Can you work these out from the model? Positions are in its coordinate system, mm. A direction names the side the tool comes from. Give positions to 0.01 mm unless a question says otherwise; leave off trailing zeros. Loops run counter-clockwise (first coordinate to the right, second up) from the corner with the lowest first, then second, coordinate; pieces in that order, holes last.
Solid Edge part; units mm, degrees
sketch "Sketch1" plane through (0, 0, 0) normal (1, 0, 0) x (0, 1, 0)
  arc A0 (2.0255, 64.2182) -> (12.0255, 54.2182) centre (2.0255, 54.2182) cw
  arc A1 (12.0255, 54.2182) -> (62.1552, -15.4154) centre (85.1165, 53.9757) ccw
  arc A2 (62.1552, -15.4154) -> (95.0255, -66.6818) centre (43.6001, -63.4831) cw
  line L0 (95.0255, -66.6818) -> (95.0255, -76.6818)
  line L1 (95.0255, -76.6818) -> (98.0468, -76.6818)
  line L2 (98.0468, -76.6818) -> (98.0468, -65.8944)
  arc A3 (62.6354, -12.4154) -> (98.0468, -65.8944) centre (43.6001, -63.4831) cw
  arc A4 (15.0228, 54.2182) -> (62.6354, -12.4154) centre (85.1165, 53.9757) ccw
  arc A5 (2.0255, 67.2155) -> (15.0228, 54.2182) centre (2.0255, 54.2182) cw
  line L3 (2.0255, 64.2182) -> (2.0255, 67.2155)
  dimension "D1" = 95.0255
  dimension "D2" = 2.0255
extrude "Protrusion1" add sketch "Sketch1" along normal blind 165
sketch "Sketch2" plane through (75, 2.0255, 65.7168) normal (0, -1, 0) x (1, 0, 0)
  line L0 (-75, 1.4986) -> (90, 1.4986)
  line L1 (90, 1.4986) -> (90, -1.4986)
  line L2 (90, -1.4986) -> (-75, -1.4986)
  line L3 (-75, -1.4986) -> (-75, 1.4986)
extrude "Extrusionsausprägung_2" add sketch "Sketch2" along normal blind 56
sketch "Sketch3" plane through (82.5, -22.9745, 67.2155) normal (0, 0, 1) x (0, 1, 0)
  circle A0 centre (-4.5, 42.5) radius 2.25
  circle A1 centre (-4.5, -42.5) radius 2.25
extrude "Cutout1" cut sketch "Sketch3" against normal through all
sketch "Sketch4" plane through (165, 28.0437, -4.7332) normal (1, 0, 0) x (0, 1, 0)
  line L0 (66.9818, -61.9486) -> (63.9818, -61.9486)
  line L1 (63.9818, -61.9486) -> (63.9818, -91.9486)
  line L2 (63.9818, -91.9486) -> (66.9818, -91.9486)
  line L3 (66.9818, -91.9486) -> (66.9818, -61.9486)
  dimension "D1" = 66.9818
  dimension "D2" = 63.9818
extrude "Protrusion2" add sketch "Sketch4" against normal up to vertex (165 mm away)
sketch "Sketch5" plane through (82.5, 95.0255, -86.6818) normal (0, 1, 0) x (1, 0, 0)
  circle A0 centre (-42.5, 0) radius 2.25
  circle A1 centre (42.5, 0) radius 2.25
  dimension "D1" = 42.5
extrude "Cutout2" cut sketch "Sketch5" against normal through all
sketch "Sketch6" plane through (0, 22.0628, -14.7332) normal (-1, 0, 0) x (0, -1, 0)
  line L0 (10.0373, 14.0132) -> (10.0373, 68.9514)
  arc A0 (-42.5155, -1.4376) -> (10.0373, 68.9514) centre (-69.9949, 73.8912) ccw
  line L1 (-42.5155, -1.4376) -> (-37.5155, -1.4376)
  line L2 (10.0373, 14.0132) -> (-37.5155, -1.4376)
  dimension "D1" = 42.5155
  dimension "D2" = 10.0373
extrude "Protrusion3" add sketch "Sketch6" against normal up to vertex (165 mm away)
sketch "Sketch7" plane through (82.5, 16.3444, -2.1232) normal (0, -0.309, -0.9511) x (0, -0.9511, 0.309)
  line L0 (-0.9588, 82.5) -> (-0.9588, 63)
  line L1 (-0.9588, 63) -> (-39.9588, 63)
  line L2 (-39.9588, 63) -> (-39.9588, 82.5)
  line L3 (-39.9588, 82.5) -> (-0.9588, 82.5)
  line L4 (-39.9588, -63) -> (-0.9588, -63)
  line L5 (-0.9588, -63) -> (-0.9588, -82.5)
  line L6 (-0.9588, -82.5) -> (-39.9588, -82.5)
  line L7 (-39.9588, -82.5) -> (-39.9588, -63)
  dimension "D1" = 0.9588
  dimension "D2" = 39.9588
extrude "Extrusionsausschnitt_3" cut sketch "Sketch7" against normal blind 2
sketch "Sketch8" plane through (82.5, 16.3444, -2.1232) normal (0, -0.309, -0.9511) x (0, -0.9511, 0.309)
  line L0 (-30.4588, 63) -> (-10.4588, 63)
  line L1 (-10.4588, 63) -> (-10.4588, 53)
  line L2 (-10.4588, 53) -> (-30.4588, 53)
  line L3 (-30.4588, 53) -> (-30.4588, 63)
  line L4 (-30.4588, -63) -> (-10.4588, -63)
  line L5 (-10.4588, -63) -> (-10.4588, -53)
  line L6 (-10.4588, -53) -> (-30.4588, -53)
  line L7 (-30.4588, -53) -> (-30.4588, -63)
  dimension "D1" = 10.4588
  dimension "D2" = 30.4588
extrude "Extrusionsausschnitt_4" cut sketch "Sketch8" against normal blind 2
sketch "Sketch9" plane through (14.75, 36.4199, -6.5432) normal (0, -0.309, -0.9511) x (1, 0, 0)
  line L0 (14.75, 10) -> (9.75, 10)
  line L1 (9.75, 10) -> (9.75, -10)
  line L2 (9.75, -10) -> (14.75, -10)
  line L3 (14.75, -10) -> (14.75, 10)
  line L4 (120.75, 10) -> (125.75, 10)
  line L5 (125.75, 10) -> (125.75, -10)
  line L6 (125.75, -10) -> (120.75, -10)
  line L7 (120.75, -10) -> (120.75, 10)
extrude "Extrusionsausschnitt_5" cut sketch "Sketch9" against normal blind 56.6903
chamfer "Fase_1" distance 0.5 angle 60 4 edges at (125, -29.7245, 67.2155) (40, -29.7245, 67.2155) (122.75, 95.0255, -86.6818) (37.75, 95.0255, -86.6818) measured on face at (25.85, -44.0812, 67.2154)
properties material "Nylon, allgemein"
(1) Suppose I cut it at D-D on z = 14.5. List the corners of the cut face in (x, y) for me.
Returned:
outline: (0, 12.03) - (165, 12.03) - (165, 27.2) - (0, 27.2) - close
(2) Suppose I cut it at A-A on x = 125. Give the number of separate pieces and of enclosed holes in the cut face, plus the area to 3 significant figures.
Returned:
separate pieces: 3
enclosed holes: 0
area: 1,390 mm2
(3) Thinking about a two-plate mould opening in X: for faces 6 (the cylindrical face through (127.146, 93.107, -87.358)), 7 (the flat face through (145.5, 50, -12)), 8 (the flat face through (81, -26, 67.215)), 9 (the flat face through (19.5, 50, -12)), which applies, pulls with the +X half, pulls with the -X half, needs draft (parallel to the pull), parting line crosses it, or undercut?
Returned:
face 6: undercut
face 7: pulls with the +X half
face 8: needs draft
face 9: pulls with the -X half
(4) Suppose I cut it at B-B on y = -44. List the corners of the cut face in (x, z) for me.
Returned:
outline: (0, 64.22) - (165, 64.22) - (165, 67.22) - (0, 67.22) - close
(5) Will these pins go through, and if not, where does the flat tip stop? P1, Ø16, axis at x = 112, z = -89, coming from the +Y side; P2, Ø2.5, axis at x = 40, z = -86.68, coming from the -Y side; P3, Ø10, axis at x = 102.5, y = 62.5, coming from the -Z side; P4, Ø4, axis at x = 117, z = -68, coming from the +Y side.
Returned:
P1: stops at y = 95.03
P2: passes through
P3: stops at z = -17.84
P4: stops at y = 98.05
(6) Please list where these lines run through material, in increasing order: probe 1 along Y at (x, z) = (125, 64.95); probe 2 along X at (y, z) = (52, -13); probe 3 along Y at (x, z) = (14, -89).
Returned:
probe 1: y = -53.97 to -29.72, -25.22 to 9.36
probe 2: x = 19.5 to 145.5
probe 3: y = 92.03 to 95.03
(7) Which directions (+Z, -Z, +X, -X, +Y, -Y) give clear straight access to the entire face, cutting with the end or side of a thin tool? Please do faces 1 (the flat face through (81, 12.026, 26)), 2 (the cylindrical face through (127.196, -27.962, 65.299)), 3 (the flat face through (19.5, 22, -3)), 4 (the flat face through (0, 50, -9)), 5 (the cylindrical face through (81.34, 87.27, -36.14)).
Returned:
face 1: -Z, +X, -X, -Y
face 2: +Z, -Z
face 3: -Z, -X
face 4: +Z, -Z, -X, +Y, -Y
face 5: +X, -X, -Y
